Answer from the drawing. Dimensions are ordinates in mm from the lowest x, y and z of the part. A direction names the side the tool comes from. Give positions to 0.01 mm unless a question says otherwise; leave off trailing zeros. Write each loop counter-clockwise with the first axis right and the second up, starting at its lowest first coordinate (ties: lowest second). Pieces come first, ordered by that corner, then holes. Notation, with made-up numbers: M 66.5,66 L 123.5,66 A24 cw 123.5,92 Z; hole C 17,65.5 d3. An arc over 180 degrees is marked long. Put each result on its own line as item: value.
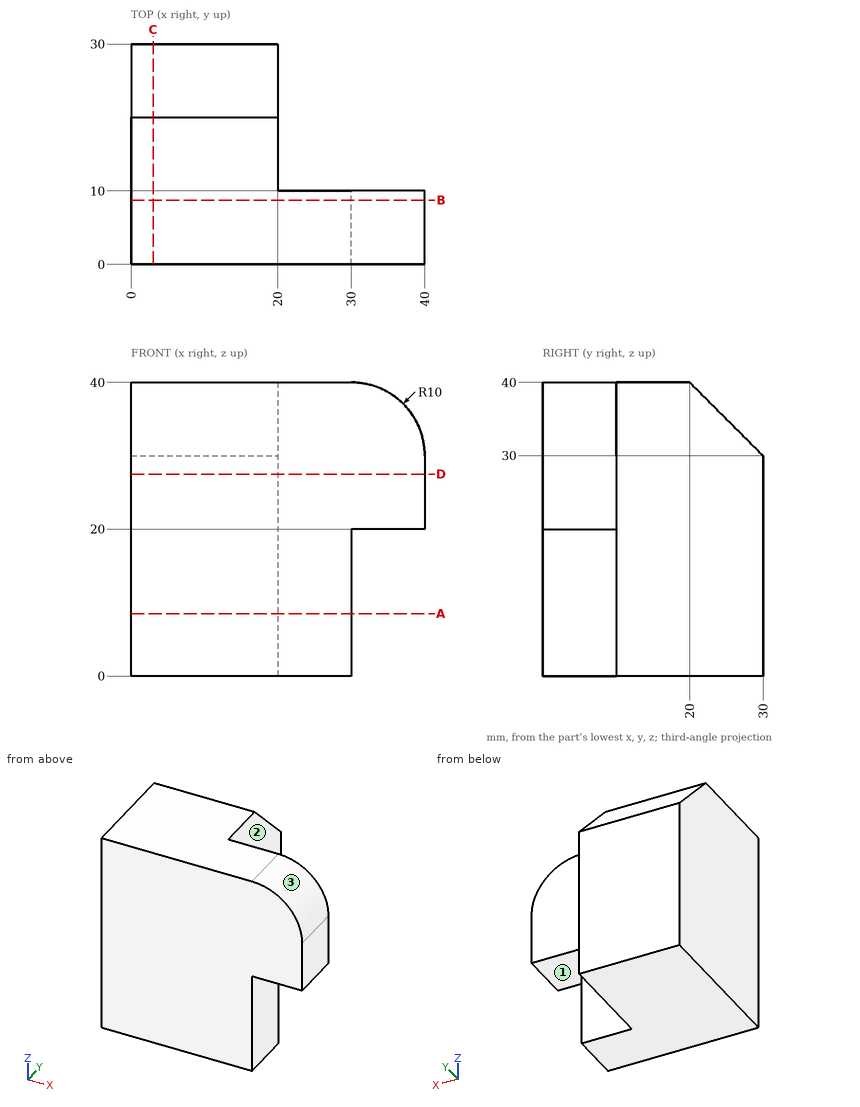
(1) Section D-D on z = 27.5 is taken. Determine the outline of the cut face in (x, y), and give its area (3 significant figures).
Result:
outline: M 0,0 L 40,0 L 40,10 L 20,10 L 20,30 L 0,30 Z
area: 800 mm²
(2) Straight lines are drawn through the part: line 1 along Y through (x, z) = (34, 29.5); line 2 along X through (y, z) = (18.5, 13.5); line 3 along X through (y, z) = (5, 11). For each, find the intervals that lie inside material, in ascending order. Write a range as from..to.
Result:
line 1: y = 0..10
line 2: x = 0..20
line 3: x = 0..30
(3) Section B-B on y = 8.75 is taken. Determine the outline of the cut face in (x, z).
Result:
outline: M 0,0 L 30,0 L 30,20 L 40,20 L 40,30 A10 ccw 30,40 L 0,40 Z
(4) Section C-C on x = 3 is taken. Determine the outline of the cut face in (y, z), and give its area (3 significant figures).
Result:
outline: M 0,0 L 30,0 L 30,30 L 20,40 L 0,40 Z
area: 1,150 mm²
(5) Section A-A on z = 8.5 is taken. Determine the outline of the cut face in (x, y), and give its area (3 significant figures).
Result:
outline: M 0,0 L 30,0 L 30,10 L 20,10 L 20,30 L 0,30 Z
area: 700 mm²
(6) Given pin 1 Ø2 at (x, y) = (33.5, 6.5) entering from +Z; pin 2 Ø3 at (x, z) = (35.5, 25.5) entering from +Y; pin 3 Ø1.5 at (y, z) = (14, 29.5) entering from +X, each flat-ended and moving along its own axis, determine where each tip first touches the part or whether it passes through.
Result:
pin 1: stops at z = 39.68
pin 2: stops at y = 10
pin 3: stops at x = 20
(7) Which of the six approach directions +Z, -Z, +X, -X, +Y, -Y give full straight-line access (tool end or side, diameter ignored) to the marked faces 1, 2 and 3?
Result:
face 1: -Z, +X, +Y, -Y
face 2: +Z, -Z, +X, +Y
face 3: +Z, +X, +Y, -Y
